from build123d import *


with BuildPart() as part:
    # Sweep1: sweep along a path in Sketch2
    with BuildLine(Plane(origin=(0, 0, 0), x_dir=(1, 0, 0), z_dir=(0, 1, 0))) as sweep1_path:
        Line((0, 0), (0, 15.631722518))
        ThreePointArc((0, 15.631722518), (3.220069275, 20.948863212), (9.423995054, 20.55881678))
        Line((9.423995054, 20.55881678), (27.143102002, 8.245243845))
        ThreePointArc((27.143102002, 8.245243845), (33.347027781, 7.855197413), (36.567097056, 13.172338107))
        Line((36.567097056, 13.172338107), (36.567097056, 53.328590127))
    # Sketch1 → Sweep1 (sweep)
    with BuildSketch(Plane.XY):
        with BuildLine():
            Line((-1.7, -1.8), (-1.7, 1.8))
            ThreePointArc((-1.7, 1.8), (0, 3.5), (1.7, 1.8))
            Line((1.7, 1.8), (1.7, -1.8))
            ThreePointArc((1.7, -1.8), (0, -3.5), (-1.7, -1.8))
        make_face()
    sweep(path=sweep1_path.line)


solid = part.part
Design review of the part built by this model. Coordinates are the model's own, in mm. A direction names the side the tool comes from. Round coordinates to 2 decimals unless told otherwise and drop trailing zeros. Write each loop counter-clockwise with the first axis right and the second up, starting at its lowest first coordinate (ties: lowest second). Pieces come first, ordered by that corner, then holes. Notation, with made-up numbers: (-6.75, -9) -> (28.25, -9) arc R19 cw to (28.25, 8) -> close; hole circle Ø3 at (16, -1.5). An arc over 180 degrees is marked (long way). One line per question, with ' | ' between items.
(1) Insertion check: P1, Ø12, axis at x = 10.5, z = -27.5, coming from the -Y side; P2, Ø1, axis at x = 6.5, y = 0.5, coming from the +Z side; P3, Ø4, axis at y = -1, z = -33, coming from the -X side. Each pin has a flat end and moves straight along its axis. Give the tip position at first contact, or say it passes through.
Result sheet:
P1: y = -3.35 | P2: z = -19.81 | P3: x = 34.87
(2) Take a section at C-C, the plane z = -42.5. State the section outline as (x, y) points, and give its area (3 significant figures).
Result sheet:
outline: (34.87, -1.8) arc R1.7 ccw to (38.27, -1.8) -> (38.27, 1.8) arc R1.7 ccw to (34.87, 1.8) -> close | area: 21.3 mm2
(3) Take a section at B-B, the plane z = -15. State how many separate pieces and enclosed holes the cut face has, and give its area (3 significant figures).
Result sheet:
separate pieces: 3 | enclosed holes: 0 | area: 80.0 mm2
(4) Draft analysis for pull direction X (two halves, no side actions). For faces 1 (the flat face through (38.267, 0, -34)), 2 (the flat face through (-1.7, 0, -8)), 3 (the flat face through (19.38, 0.03, -15.71)), state which applies: released by +X, released by -X, zero draft, split by the parting line, or undercut.
Result sheet:
face 1: released by +X | face 2: released by -X | face 3: undercut
(5) Take a section at D-D, the plane y = 2.5. State the section outline as (x, z) points.
Result sheet:
outline: (-1.55, -15.63) arc R7.55 ccw to (10.31, -21.83) -> (28.03, -9.52) arc R4.45 cw to (35.02, -13.17) -> (35.02, -53.33) -> (38.12, -53.33) -> (38.12, -13.17) arc R7.55 ccw to (26.26, -6.97) -> (8.54, -19.29) arc R4.45 cw to (1.55, -15.63) -> (1.55, 0) -> (-1.55, 0) -> close
(6) Machinability: for faces 4 (the cylindrical face through (36.6, -3.5, -33.5)), 5 (the flat face through (17.44, -0.03, -12.92)), 6 (the flat face through (34.867, 0, -34)), 7 (the cylindrical face through (36.5, 3.5, -33.5)), 8 (the cylindrical face through (0, -3.5, -7.9)), which of the approach directions +Z, -Z, +X, -X, +Y, -Y give a long, thin tool a straight path to every point of the face, cutting with its end or side? Answer none if there is none.
Result sheet:
face 4: -Z, -Y | face 5: +Z, +Y, -Y | face 6: -Z, +Y, -Y | face 7: -Z, +Y | face 8: +Z, -Y
(7) Wall thickness on line 1 (X direction, y = 1.5, z = -30); line 2 (Z direction, x = 8, y = 3.25); line 3 (Y direction, x = 20.5, z = -12): over which ranges is each line inside the solid? List them lowest first. Write a range as [from, to].
Result sheet:
line 1: [34.87, 38.27] | line 2: [-22.22, -20.34] | line 3: [-3.35, 3.35]
(8) Take a section at A-A, the plane y = -0.75. State the section outline as (x, z) points.
Result sheet:
outline: (-1.7, -15.63) arc R7.7 ccw to (10.39, -21.95) -> (28.11, -9.64) arc R4.3 cw to (34.87, -13.17) -> (34.87, -53.33) -> (38.27, -53.33) -> (38.27, -13.17) arc R7.7 ccw to (26.17, -6.85) -> (8.45, -19.16) arc R4.3 cw to (1.7, -15.63) -> (1.7, 0) -> (-1.7, 0) -> close
